Geometry: final body of the model. Coordinates: model frame, mm. A direction names the side the tool comes from. Round coordinates to 2 decimals unless told otherwise and drop trailing zeros. Order: outer loops, then holes, each group sorted by start corner. A loop starts at its lowest first (then second) coordinate and runs counter-clockwise, first axis right, second up. Notation, with made-up numbers: M 52,-33.5 L 83,-33.5 A15 cw 83,-9.5 Z; hole C -34.5,-5 d6. An arc over 180 degrees is marked long. Put each result on its own line as item: value. Start each with the question number.
1) Access query for faces 1 (the flat face through (50, 8, 65)), 2 (the flat face through (53, 10, 15)), 3 (the flat face through (50, 18, -5)), 4 (the flat face through (40, 72, 2.5)), 5 (the flat face through (-55, 8, -10.12)). Directions: +Z, -Z, +X, -X, +Y, -Y. A direction counts if a zero-diameter tool reaches every point of the face in a straight line with its end or side. Return the directions, or none.
2) Material intervals for probe 1 along Z at (x, y) = (62.5, 6.45); probe 2 along Y at (x, z) = (11.5, 1); probe 3 along Z at (x, y) = (-55, 7.9), sorted ascending. Write a range as [from, to].
3) Section A-A, the plane y = 106. Return loops of the section in (x, z).
4) Section B-B, the plane x = 27.5. Count the separate pieces of the cut face and the enclosed holes in it, then the cut area to 4 significant figures.
5) Draft query along Y for faces 6 (the flat face through (27, 136, 0)), 7 (the flat face through (39, 89, 15)), 8 (the flat face through (20, 5, 14)). Return one class per face: pulls with the +Y half, pulls with the -Y half, needs draft (parallel to the pull), parting line crosses it, or undercut.
6) First-contact query: P1, Ø5, axis at x = 49, y = 48, coming from the -Z side; P2, Ø12, axis at x = -0.5, y = 69.5, coming from the -Z side; P3, Ø2, axis at x = 22.5, y = 85.5, coming from the +Z side. Flat tips, straight axial feed; report the tip coordinate or a pass-through.
7) Section D-D, the plane z = -39. Return loops of the section in (x, y).
from build123d import *

# Parameters (mm, degrees)
PAD_DEPTH       = 30
SKETCH001_W     = 10
SKETCH001_H     = 150
PAD001_DEPTH    = 180
SKETCH002_W     = 25
SKETCH002_H     = 150
PAD002_DEPTH    = 153
SKETCH003_W     = 5
SKETCH003_H     = 3
SKETCH003_W_2   = 11
SKETCH003_H_2   = 2
POCKET_DEPTH    = 150
SKETCH006_W     = 153
SKETCH006_H     = 50
POCKET001_DEPTH = 35
SKETCH007_W     = 50
SKETCH007_H     = 50
SKETCH007_W_2   = 45
POCKET002_DEPTH = 35
SKETCH004_R     = 2
POCKET003_DEPTH = 10.001
SKETCH008_W     = 25
SKETCH008_H     = 25
SKETCH008_W_2   = 20
SKETCH008_W_3   = 5
SKETCH008_H_2   = 50
POCKET004_DEPTH = 150
SKETCH009_W     = 5
SKETCH009_H     = 150
POCKET005_DEPTH = 200
SKETCH010_W     = 20
SKETCH010_H     = 30
POCKET006_DEPTH = 5
SKETCH011_W     = 70
SKETCH011_H     = 30
POCKET007_DEPTH = 128
SKETCH012_W     = 65
SKETCH012_H     = 150
POCKET008_DEPTH = 5
SKETCH013_W     = 5
SKETCH013_H     = 50
POCKET009_DEPTH = 20
SKETCH014_W     = 20
SKETCH014_H     = 50
POCKET010_DEPTH = 5
SKETCH015_W     = 17
SKETCH015_H     = 30
POCKET011_DEPTH = 6
SKETCH016_W     = 5
SKETCH016_H     = 50
PAD003_DEPTH    = 30
SKETCH017_R     = 2
POCKET012_DEPTH = 5
SKETCH018_W     = 6
SKETCH018_H     = 17
POCKET013_DEPTH = 30


with BuildPart() as part:
    # Sketch → Pad (new body)
    with BuildSketch(Plane.XY):
        Polygon((-75, 0), (75, 0), (75, 163), (-65, 163), (-65, 153), (55, 153), (55, 151), (-65, 151), (-65, 121), (55, 121), (55, 119), (-65, 119), (-65, 89), (55, 89), (55, 87), (-65, 87), (-65, 57), (55, 57), (55, 55), (-65, 55), (-65, 30), (55, 30), (55, 27), (25, 27), (25, 10), (-75, 10), align=None)
    extrude(amount=PAD_DEPTH)

    # Sketch001 (on Face2 of Pad) → Pad001 (join)
    with BuildSketch(Plane.YZ.offset(75)):
        with Locations((5, 15)):
            Rectangle(SKETCH001_W, SKETCH001_H)
    extrude(amount=-PAD001_DEPTH)

    # Sketch002 (on Face10 of Pad001) → Pad002 (join)
    with BuildSketch(Plane(origin=(0, 10, 0), x_dir=(-1, 0, 0), z_dir=(0, 1, 0))):
        with Locations((-62.5, 15)):
            Rectangle(SKETCH002_W, SKETCH002_H)
    extrude(amount=PAD002_DEPTH)

    # Sketch003 (on Face14 of Pad002) → Pocket (cut)
    with BuildSketch(Plane.XY.offset(90)):
        with Locations((52.5, 28.5)):
            Rectangle(SKETCH003_W, SKETCH003_H)
        with Locations((55.5, 56)):
            Rectangle(SKETCH003_W_2, SKETCH003_H_2)
        with Locations((55.5, 88)):
            Rectangle(SKETCH003_W_2, SKETCH003_H_2)
        with Locations((55.5, 120)):
            Rectangle(SKETCH003_W_2, SKETCH003_H_2)
        with Locations((55.5, 152)):
            Rectangle(SKETCH003_W_2, SKETCH003_H_2)
    extrude(amount=-POCKET_DEPTH, mode=Mode.SUBTRACT)

    # Sketch006 → Pocket001 (cut)
    with BuildSketch(Plane(origin=(49, 0, 0), x_dir=(0, -1, 0), z_dir=(-1, 0, 0))):
        with Locations((-86.5, 65)):
            Rectangle(SKETCH006_W, SKETCH006_H)
        with Locations((-86.5, -35)):
            Rectangle(SKETCH006_W, SKETCH006_H)
    extrude(amount=-POCKET001_DEPTH, mode=Mode.SUBTRACT)

    # Sketch007 → Pocket002 (cut)
    with BuildSketch(Plane(origin=(0, 10, 0), x_dir=(-1, 0, 0), z_dir=(0, 1, 0))):
        with Locations((-5, 65)):
            Rectangle(SKETCH007_W, SKETCH007_H)
        with Locations((62.5, 65)):
            Rectangle(SKETCH007_W_2, SKETCH007_H)
        with Locations((-5, -35)):
            Rectangle(SKETCH007_W, SKETCH007_H)
        with Locations((62.5, -35)):
            Rectangle(SKETCH007_W_2, SKETCH007_H)
    extrude(amount=-POCKET002_DEPTH, mode=Mode.SUBTRACT)

    # Sketch004 (on Face13 of Pocket) → Pocket003 (cut, through all)
    with BuildSketch(Plane(origin=(0, 10, 0), x_dir=(-1, 0, 0), z_dir=(0, 1, 0))):
        with Locations((-62.5, 80)):
            Circle(SKETCH004_R)
        with Locations((30, 80)):
            Circle(SKETCH004_R)
        with Locations((95, 80)):
            Circle(SKETCH004_R)
        with Locations((-62.5, -50)):
            Circle(SKETCH004_R)
        with Locations((30, -50)):
            Circle(SKETCH004_R)
        with Locations((95, -50)):
            Circle(SKETCH004_R)
    extrude(amount=-POCKET003_DEPTH, mode=Mode.SUBTRACT)

    # Sketch008 (on Face100 of Pocket003) → Pocket004 (cut)
    with BuildSketch(Plane(origin=(-65, 0, 0), x_dir=(0, -1, 0), z_dir=(-1, 0, 0))):
        with Locations((-136, 15)):
            Rectangle(SKETCH008_W, SKETCH008_H)
        with Locations((-104, 15)):
            Rectangle(SKETCH008_W, SKETCH008_H)
        with Locations((-72, 15)):
            Rectangle(SKETCH008_W, SKETCH008_H)
        with Locations((-42.5, 15)):
            Rectangle(SKETCH008_W_2, SKETCH008_H)
        with Locations((-160.5, 15)):
            Rectangle(SKETCH008_W_3, SKETCH008_H_2)
    extrude(amount=-POCKET004_DEPTH, mode=Mode.SUBTRACT)

    # Sketch009 (on Face20 of Pocket004) → Pocket005 (cut)
    with BuildSketch(Plane(origin=(-105, 0, 0), x_dir=(0, -1, 0), z_dir=(-1, 0, 0))):
        with Locations((-2.5, 15)):
            Rectangle(SKETCH009_W, SKETCH009_H)
    extrude(amount=-POCKET005_DEPTH, mode=Mode.SUBTRACT)

    # Sketch010 (on Face66 of Pocket005) → Pocket006 (cut)
    with BuildSketch(Plane(origin=(0, 10, 0), x_dir=(-1, 0, 0), z_dir=(0, 1, 0))):
        with Locations((65, 15)):
            Rectangle(SKETCH010_W, SKETCH010_H)
    extrude(amount=-POCKET006_DEPTH, mode=Mode.SUBTRACT)

    # Sketch011 (on Face39 of Pocket006) → Pocket007 (cut)
    with BuildSketch(Plane(origin=(0, 158, 0), x_dir=(-1, 0, 0), z_dir=(0, 1, 0))):
        with Locations((30, 15)):
            Rectangle(SKETCH011_W, SKETCH011_H)
    extrude(amount=-POCKET007_DEPTH, mode=Mode.SUBTRACT)

    # Sketch012 (on Face56 of Pocket007) → Pocket008 (cut)
    with BuildSketch(Plane(origin=(0, 10, 0), x_dir=(-1, 0, 0), z_dir=(0, 1, 0))):
        with Locations((72.5, 15)):
            Rectangle(SKETCH012_W, SKETCH012_H)
    extrude(amount=-POCKET008_DEPTH, mode=Mode.SUBTRACT)

    # Sketch013 (on Face14 of Pocket008) → Pocket009 (cut)
    with BuildSketch(Plane(origin=(30, 0, 0), x_dir=(0, -1, 0), z_dir=(-1, 0, 0))):
        with Locations((-7.5, -35)):
            Rectangle(SKETCH013_W, SKETCH013_H)
        with Locations((-7.5, 65)):
            Rectangle(SKETCH013_W, SKETCH013_H)
    extrude(amount=-POCKET009_DEPTH, mode=Mode.SUBTRACT)

    # Sketch014 (on Face3 of Pocket009) → Pocket010 (cut)
    with BuildSketch(Plane.XZ.offset(-5)):
        with Locations((-30, -35)):
            Rectangle(SKETCH014_W, SKETCH014_H)
        with Locations((-30, 65)):
            Rectangle(SKETCH014_W, SKETCH014_H)
    extrude(amount=-POCKET010_DEPTH, mode=Mode.SUBTRACT)

    # Sketch015 (on Face79 of Pocket010) → Pocket011 (cut)
    with BuildSketch(Plane(origin=(50, 0, 0), x_dir=(0, -1, 0), z_dir=(-1, 0, 0))):
        with Locations((-18.5, 15)):
            Rectangle(SKETCH015_W, SKETCH015_H)
    extrude(amount=-POCKET011_DEPTH, mode=Mode.SUBTRACT)

    # Sketch016 (on Face18 of Pocket011) → Pad003 (join)
    with BuildSketch(Plane(origin=(-40, 0, 0), x_dir=(0, -1, 0), z_dir=(-1, 0, 0))):
        with Locations((-7.5, 14.879722)):
            Rectangle(SKETCH016_W, SKETCH016_H)
    extrude(amount=PAD003_DEPTH)

    # Sketch017 (on Face78 of Pad003) → Pocket012 (cut)
    with BuildSketch(Plane(origin=(0, 10, 0), x_dir=(-1, 0, 0), z_dir=(0, 1, 0))):
        with Locations((55, 30)):
            Circle(SKETCH017_R)
        with Locations((55, 0)):
            Circle(SKETCH017_R)
    extrude(amount=-POCKET012_DEPTH, mode=Mode.SUBTRACT)

    # Sketch018 (on Face84 of Pocket012) → Pocket013 (cut)
    with BuildSketch(Plane.XY.offset(30)):
        with Locations((28, 18.5)):
            Rectangle(SKETCH018_W, SKETCH018_H)
    extrude(amount=-POCKET013_DEPTH, mode=Mode.SUBTRACT)


solid = part.part
Result sheet:
1. face 1: +Z, -X, +Y, -Y
1. face 2: none
1. face 3: -Z, -X, +Y
1. face 4: +X, -X
1. face 5: -Z, -X, +Y, -Y
2. probe 1: z = [-60, -52], [-48, 78], [82, 90]
2. probe 2: y = [5, 10], [30, 55], [57, 87], [89, 119], [121, 151], [153, 158]
2. probe 3: z = [-10.12, -2], [2, 28], [32, 39.88]
3. outline: M 5,0 L 50,0 L 50,-10 L 75,-10 L 75,2.5 L 5,2.5 Z; M 5,27.5 L 75,27.5 L 75,40 L 50,40 L 50,30 L 5,30 Z
4. separate pieces: 6
4. enclosed holes: 4
4. area: 1,475 mm2
5. face 6: needs draft
5. face 7: undercut
5. face 8: pulls with the -Y half
6. P1: stops at z = -10
6. P2: stops at z = 0
6. P3: stops at z = 30
7. outline: M 50,5 L 75,5 L 75,10 L 50,10 Z
